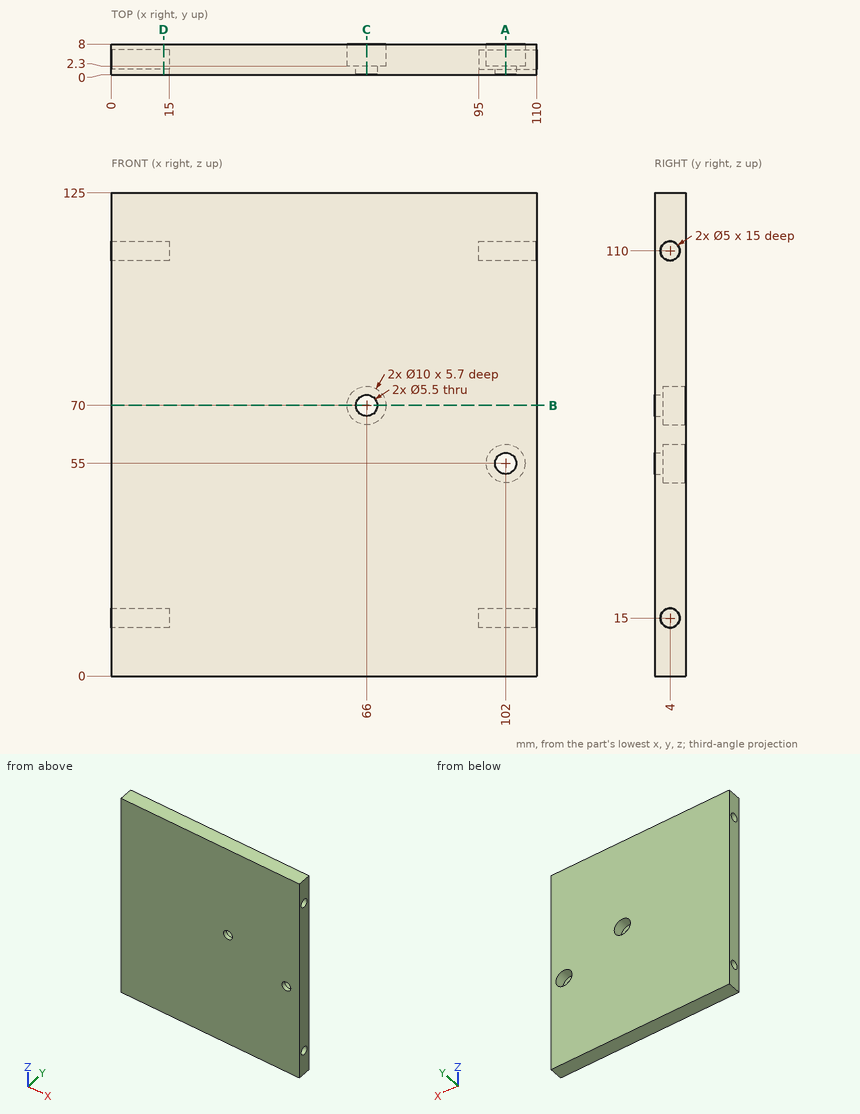
The figure shows three views and two pictorial views of one solid part (mm, origin at its lowest corner). Answer the questions. Coordinates: 2 decimals unless noted, no trailing zeros. Write each loop counter-clockwise with the first axis right and the second up, starting at its lowest first coordinate (ties: lowest second). Pieces come first, ordered by that corner, then holes.
1. The part is cut by section B-B, the plane z = 70. Write down the section's boundary in (x, y).
Results list:
outline: (0, 0) - (63.25, 0) - (63.25, 2.3) - (61, 2.3) - (61, 8) - (0, 8) - close; (68.75, 0) - (110, 0) - (110, 8) - (71, 8) - (71, 2.3) - (68.75, 2.3) - close
2. Consider line 1 along X through (y, z) = (4.5, 70.5); line 2 along Z through (x, y) = (102, 0.85); line 3 along Z through (x, y) = (7, 2.5). Determine where each line is inside the solid, lowest interval first.
Results list:
line 1: x = 0 to 61.03, 70.97 to 110
line 2: z = 0 to 52.25, 57.75 to 125
line 3: z = 0 to 13, 17 to 108, 112 to 125
3. The part is cut by section A-A, the plane x = 102. Write down the section's boundary in (y, z).
Results list:
outline: (0, 0) - (8, 0) - (8, 50) - (2.3, 50) - (2.3, 52.25) - (0, 52.25) - close; (0, 57.75) - (2.3, 57.75) - (2.3, 60) - (8, 60) - (8, 125) - (0, 125) - close; hole circle Ø5 at (4, 15); hole circle Ø5 at (4, 110)
4. The part is cut by section C-C, the plane x = 66. Write down the section's boundary in (y, z).
Results list:
outline: (0, 0) - (8, 0) - (8, 65) - (2.3, 65) - (2.3, 67.25) - (0, 67.25) - close; (0, 72.75) - (2.3, 72.75) - (2.3, 75) - (8, 75) - (8, 125) - (0, 125) - close
5. Flat-ended cylindrical pins translate along their axes: pin 1 (6 mm diameter, centred on x = 77, z = 13, fed in from -Y); pin 2 (1.5 mm diameter, centred on y = 5, z = 16, fed in from -X); pin 3 (4 mm diameter, centred on y = 4, z = 110, fed in from +X); pin 4 (8 mm diameter, centred on x = 66, z = 70, fed in from +Y). Find the tip coordinate at first contact, or state that the pin passes through.
Results list:
pin 1: stops at y = 0
pin 2: stops at x = 15
pin 3: stops at x = 95
pin 4: stops at y = 2.3
6. The part is cut by section D-D, the plane x = 13.5. Write down the section's boundary in (y, z).
Results list:
outline: (0, 0) - (8, 0) - (8, 125) - (0, 125) - close; hole circle Ø5 at (4, 15); hole circle Ø5 at (4, 110)
